Autodesk Inventor part; units mm, degrees
ref_plane "YZ Plane" through (0, 0, 0) normal (1, 0, 0) x (0, 1, 0)
ref_plane "XZ Plane" through (0, 0, 0) normal (0, 1, 0) x (-1, 0, 0)
ref_plane "XY Plane" through (0, 0, 0) normal (0, 0, 1) x (1, 0, 0)
sketch "Sketch1" plane through (0, 0, 0) normal (1, 0, 0) x (0, 1, 0)
  line L0 (-787.4, -234.95) -> (787.4, -234.95)
  line L1 (787.4, -234.95) -> (787.4, 234.95)
  line L2 (787.4, 234.95) -> (-787.4, 234.95)
  line L3 (-787.4, 234.95) -> (-787.4, -234.95)
  line L4 (-787.4, -234.95) -> (787.4, 234.95) construction
  line L5 (787.4, -234.95) -> (-787.4, 234.95) construction
  point P0 (0, 0)
  dimension "d0" = 1574.8
  dimension "d1" = 469.9
extrude "Extrusion1" add sketch "Sketch1" along normal blind 19.05
sketch "Sketch2" plane through (0, 0, 0) normal (-1, 0, 0) x (0, 0, 1)
  circle A0 centre (163.83, -482.6) radius 38.1
  line L0 (234.95, 787.4) -> (234.95, -787.4)
  line L1 (234.95, -787.4) -> (-234.95, -787.4)
  point P0 (0, 0)
  point P1 (0, 0)
  dimension "d5" = 76.2
  dimension "d8" = 71.12
  dimension "d9" = 304.8
extrude "Extrusion2" cut sketch "Sketch2" against normal blind 25.4
properties part number "back board (for assembly)"
Verification items for the finished model (mm, model axes). Give positions to 0.01 mm unless a question says otherwise; leave off trailing zeros. Order: outer loops, then holes, each group sorted by start corner. A loop starts at its lowest first (then second) coordinate and runs counter-clockwise, first axis right, second up. Notation, with made-up numbers: M 2.5,49 L 29.5,49 A17 cw 29.5,64 Z; hole C -28.75,-27 d2. An arc over 180 degrees is marked long. Return JSON: item names as keys, results as strings. Group by question number.
1) Go/stop test with a flat-tipped pin: pin 1 Ø12 at (y, z) = (-615.5, -118.5) entering from -X. Record where the tip stops, or that it passes through.
2) Section check A-A on y = -482.6. Record the cut outline in (x, z), and give its area (3 significant figures).
3) Mould release check, pull along Z, two halves, no side actions. Record for faces 1 (the face through (19.05, -11, 3)), 2 (the face through (9.4, -519.8, 155.6)): pulls with the +Z half, pulls with the -Z half, needs draft (parallel to the pull), parting line crosses it, or undercut.
4) Section check B-B on z = 163.83. Record the cut outline in (x, y), and give its area (3 significant figures).
5) Scan lines: line 1 (Y direction, x = 16.5, z = 160); line 2 (Y direction, x = 6.5, z = 163.83). Record each from-to range of solid material in increasing order.
Answer block:
{
 "1": {"pin 1": "stops at x = 0"},
 "2": {"outline": "M 0,-234.95 L 19.05,-234.95 L 19.05,125.73 L 0,125.73 Z; M 0,201.93 L 19.05,201.93 L 19.05,234.95 L 0,234.95 Z", "area": "7,500 mm^2"},
 "3": {"face 1": "needs draft", "face 2": "undercut"},
 "4": {"outline": "M 0,-787.4 L 19.05,-787.4 L 19.05,-520.7 L 0,-520.7 Z; M 0,-444.5 L 19.05,-444.5 L 19.05,787.4 L 0,787.4 Z", "area": "28,500 mm^2"},
 "5": {"line 1": "y = -787.4 to -520.51, -444.69 to 787.4", "line 2": "y = -787.4 to -520.7, -444.5 to 787.4"}
}
